from build123d import *

# Parameters (mm, degrees)
SKICA1_W                 = 184
SKICA1_H                 = 121
P_IDAT_VYSUNUT_M1_DEPTH  = 2
SKICA2_W                 = 32
SKICA2_H                 = 10
ODEBRAT_VYSUNUT_M1_DEPTH = 3
SKICA3_W                 = 35
SKICA3_H                 = 50
ODEBRAT_VYSUNUT_M2_DEPTH = 10
SKICA5_W                 = 90
SKICA5_H                 = 60
ODEBRAT_VYSUNUT_M3_DEPTH = 10
SKICA6_W                 = 94
SKICA6_H                 = 64
SKICA6_W_2               = 90
SKICA6_H_2               = 60
P_IDAT_VYSUNUT_M2_DEPTH  = 10
ODEBRAT_VYSUNUT_M4_DEPTH = 93.5
P_IDAT_VYSUNUT_M3_DEPTH  = 64
SKICA9_W                 = 89.439473795
SKICA9_H                 = 64
P_IDAT_VYSUNUT_M4_DEPTH  = 1.5
ODEBRAT_VYSUNUT_M5_DEPTH = 93.5
P_IDAT_VYSUNUT_M5_DEPTH  = 0.75
LINPOLE1_COUNT           = 2
LINPOLE1_PITCH           = 15
LINPOLE1_COL_COUNT       = 2
LINPOLE1_COL_PITCH       = 15
SKICA12_W                = 1
SKICA12_H                = 8
ODEBRAT_VYSUNUT_M6_DEPTH = 31.5


with BuildPart() as part:
    # Skica1 → Přidat vysunutím1 (new body)
    with BuildSketch(Plane(origin=(0, 0, 0), x_dir=(1, 0, 0), z_dir=(0, 1, 0))):
        Rectangle(SKICA1_W, SKICA1_H)
    extrude(amount=P_IDAT_VYSUNUT_M1_DEPTH)

    # Skica2 → Odebrat vysunutím1 (cut)
    with BuildSketch(Plane(origin=(0, 2, 0), x_dir=(1, 0, 0), z_dir=(0, 1, 0))):
        with Locations((-44, 55.5)):
            Rectangle(SKICA2_W, SKICA2_H)
        with Locations((-44, -55.5)):
            Rectangle(SKICA2_W, SKICA2_H)
    extrude(amount=-ODEBRAT_VYSUNUT_M1_DEPTH, mode=Mode.SUBTRACT)

    # Skica3 → Odebrat vysunutím2 (cut)
    with BuildSketch(Plane(origin=(0, 2, 0), x_dir=(1, 0, 0), z_dir=(0, 1, 0))):
        with Locations((-74.5, 0)):
            Rectangle(SKICA3_W, SKICA3_H)
    extrude(amount=-ODEBRAT_VYSUNUT_M2_DEPTH, mode=Mode.SUBTRACT)

    # Skica5 → Odebrat vysunutím3 (cut)
    with BuildSketch(Plane(origin=(0, 2, 0), x_dir=(1, 0, 0), z_dir=(0, 1, 0))):
        with Locations((38, 0)):
            Rectangle(SKICA5_W, SKICA5_H)
    extrude(amount=-ODEBRAT_VYSUNUT_M3_DEPTH, mode=Mode.SUBTRACT)

    # Skica6 → Přidat vysunutím2 (add)
    with BuildSketch(Plane(origin=(0, 2, 0), x_dir=(1, 0, 0), z_dir=(0, 1, 0))):
        with Locations((38, 0)):
            Rectangle(SKICA6_W, SKICA6_H)
        with Locations((38, 0)):
            Rectangle(SKICA6_W_2, SKICA6_H_2, mode=Mode.SUBTRACT)
    extrude(amount=P_IDAT_VYSUNUT_M2_DEPTH)

    # Skica7 → Odebrat vysunutím4 (cut, through all)
    with BuildSketch(Plane.XY.offset(32)):
        Polygon((-9, 2), (-1.997924618, 12), (-9, 12), align=None)
    extrude(amount=-ODEBRAT_VYSUNUT_M4_DEPTH, mode=Mode.SUBTRACT)

    # Skica8 → Přidat vysunutím3 (add)
    with BuildSketch(Plane.XY.offset(32)):
        Polygon((-1.997924618, 12), (-4.439473795, 12), (-11.441549178, 2), (-9, 2), align=None)
    extrude(amount=-P_IDAT_VYSUNUT_M3_DEPTH)

    # Skica9 → Přidat vysunutím4 (add)
    with BuildSketch(Plane(origin=(0, 12, 0), x_dir=(1, 0, 0), z_dir=(0, 1, 0))):
        with Locations((40.280263103, 0)):
            Rectangle(SKICA9_W, SKICA9_H)
    extrude(amount=P_IDAT_VYSUNUT_M4_DEPTH)

    # Skica10 → Odebrat vysunutím5 (cut, through all)
    with BuildSketch(Plane.XY.offset(32)):
        Polygon((-4.439473795, 12), (-3.389162488, 13.5), (-4.439473795, 13.5), align=None)
    extrude(amount=-ODEBRAT_VYSUNUT_M5_DEPTH, mode=Mode.SUBTRACT)

    # Skica11 → Přidat vysunutím5 (add, symmetric)
    with BuildSketch(Plane.XY):
        Polygon((83, 12), (-1.997924618, 12), (-7, 4.856296013), (-7, 0), (83, 0), align=None)
    p_idat_vysunut_m5 = extrude(amount=P_IDAT_VYSUNUT_M5_DEPTH, both=True)

    # LinPole1: Přidat vysunutím5 ×2
    with Locations(*[(0, 0, i * LINPOLE1_PITCH) for i in range(1, LINPOLE1_COUNT)]):
        add(p_idat_vysunut_m5)

    # LinPole1 col: Přidat vysunutím5 ×2
    with Locations(*[(0, 0, -i * LINPOLE1_COL_PITCH) for i in range(1, LINPOLE1_COL_COUNT)]):
        add(p_idat_vysunut_m5)

    # Skica12 → Odebrat vysunutím6 (cut)
    with BuildSketch(Plane.XY.offset(15.75)):
        with Locations((8.5, 4)):
            Rectangle(SKICA12_W, SKICA12_H)
        with Locations((34.5, 4)):
            Rectangle(SKICA12_W, SKICA12_H)
        with Locations((60.5, 4)):
            Rectangle(SKICA12_W, SKICA12_H)
    extrude(amount=-ODEBRAT_VYSUNUT_M6_DEPTH, mode=Mode.SUBTRACT)


solid = part.part
Read the model definition and answer for the solid it produces. Units are mm, in the model's axes. Round coordinates to 2 decimals unless told otherwise and drop trailing zeros. Loops run counter-clockwise (first coordinate to the right, second up) from the corner with the lowest first, then second, coordinate; pieces in that order, holes last.
Q1. Each of these flat-tipped pins is pushed along its axis until it touches: pin 1 (0.8 mm diameter, centred on y = 4.5, z = 15.5, fed in from +X); pin 2 (8 mm diameter, centred on y = 10, z = -26, fed in from -X); pin 3 (1.6 mm diameter, centred on x = -48.5, y = 1, fed in from +Z); pin 4 (8 mm diameter, centred on y = 10, z = 38.5, fed in from -X). Where does it stop, or does it pass through?
Q2. Determine the mould class of faces 1 (the face through (36, 8, -32)), 2 (the face through (-4.534, 8.378, -7.406)), 3 (the face through (83, 6, 8)) for opening direction X: released by +X, released by -X, zero draft, split by the parting line, or undercut.
Q3. Section C-C on y = 10 is taken. Write down the section's boundary in (x, z), and give its area (3 significant figures).
Q4. Consider probe 1 along Z at (x, y) = (77.5, 9.5); probe 2 along Z at (x, y) = (4.5, 1); probe 3 along Y at (x, z) = (-2.5, 47). Determine where each line is inside the solid, lowest interval first.
Q5. Section B-B on x = 77.5 is taken. Write down the section's boundary in (y, z).
Q6. Section D-D on z = -18 is taken. Write down the section's boundary in (x, y), and give its area (3 significant figures).
Q7. Section A-A on z = -52.5 is taken. Write down the section's boundary in (x, y), and give its area (3 significant figures).
Output:
1. pin 1: stops at x = 85
1. pin 2: stops at x = -8.64
1. pin 3: stops at z = 50.5
1. pin 4: passes through
2. face 1: zero draft
2. face 2: undercut
2. face 3: undercut
3. outline: (-5.84, -32) - (85, -32) - (85, 32) - (-5.84, 32) - close; hole (-3.4, -30) - (83, -30) - (83, -15.75) - (-3.4, -15.75) - close; hole (-3.4, -14.25) - (83, -14.25) - (83, -0.75) - (-3.4, -0.75) - close; hole (-3.4, 0.75) - (83, 0.75) - (83, 14.25) - (-3.4, 14.25) - close; hole (-3.4, 15.75) - (83, 15.75) - (83, 30) - (-3.4, 30) - close
3. area: 1,020 mm2
4. probe 1: z = -32 to -30, -15.75 to -14.25, -0.75 to 0.75, 14.25 to 15.75, 30 to 32
4. probe 2: z = -60.5 to -30, -15.75 to -14.25, -0.75 to 0.75, 14.25 to 15.75, 30 to 60.5
4. probe 3: y = 0 to 2
5. outline: (0, -60.5) - (2, -60.5) - (2, -32) - (13.5, -32) - (13.5, 32) - (2, 32) - (2, 60.5) - (0, 60.5) - (0, 30) - (12, 30) - (12, 15.75) - (0, 15.75) - (0, 14.25) - (12, 14.25) - (12, 0.75) - (0, 0.75) - (0, -0.75) - (12, -0.75) - (12, -14.25) - (0, -14.25) - (0, -15.75) - (12, -15.75) - (12, -30) - (0, -30) - close
6. outline: (-57, 0) - (-7, 0) - (-7, 4.86) - (-2, 12) - (83, 12) - (83, 0) - (92, 0) - (92, 2) - (85, 2) - (85, 13.5) - (-3.39, 13.5) - (-11.44, 2) - (-57, 2) - close
6. area: 299 mm2
7. outline: (-92, 0) - (-60, 0) - (-60, 2) - (-92, 2) - close; (-28, 0) - (92, 0) - (92, 2) - (-28, 2) - close
7. area: 304 mm2
